```python
from build123d import *

# Parameters (mm, degrees)
F0_R     = 10.9982
F1_DEPTH = 7


with BuildPart() as f1:
    # F0 (on Top) → F1 (new body)
    with BuildSketch(Plane.XY):
        with BuildLine():
            ThreePointArc((12.246776, 8.324618), (12.094028, 24.483764), (14.8082, 40.414069))
            ThreePointArc((14.8082, 40.414069), (0, 55.222269), (-14.8082, 40.414069))
            ThreePointArc((-14.8082, 40.414069), (-12.094028, 24.483764), (-12.246776, 8.324618))
            ThreePointArc((-12.246776, 8.324618), (-12.824277, 7.4041), (-13.332719, 6.44371))
            ThreePointArc((-13.332719, 6.44371), (-27.250576, -1.768146), (-42.40371, -7.382757))
            ThreePointArc((-42.40371, -7.382757), (-47.823888, -27.611134), (-27.59551, -33.031312))
            ThreePointArc((-27.59551, -33.031312), (-15.156548, -22.715618), (-1.085942, -14.768328))
            ThreePointArc((-1.085942, -14.768328), (0, -14.8082), (1.085942, -14.768328))
            ThreePointArc((1.085942, -14.768328), (15.156548, -22.715618), (27.59551, -33.031312))
            ThreePointArc((27.59551, -33.031312), (47.823888, -27.611134), (42.40371, -7.382757))
            ThreePointArc((42.40371, -7.382757), (27.250576, -1.768146), (13.332719, 6.44371))
            ThreePointArc((13.332719, 6.44371), (12.824277, 7.4041), (12.246776, 8.324618))
        make_face()
        with Locations((-34.99961, -20.207034)):
            Circle(F0_R, mode=Mode.SUBTRACT)
        with Locations((34.99961, -20.207034)):
            Circle(F0_R, mode=Mode.SUBTRACT)
        Circle(F0_R, mode=Mode.SUBTRACT)
        with BuildLine():
            ThreePointArc((-10.9982, 40.414069), (0, 51.412269), (10.9982, 40.414069))
            ThreePointArc((10.9982, 40.414069), (0, 29.415869), (-10.9982, 40.414069))
        make_face(mode=Mode.SUBTRACT)
    extrude(amount=F1_DEPTH)


solid = f1.part
```
Geometry check sheet. Reference: the model listing, model coordinates, mm. A direction names the side the tool comes from. Coordinates: 2 decimals unless noted, no trailing zeros. Order: outer loops, then holes, each group sorted by start corner. A loop starts at its lowest first (then second) coordinate and runs counter-clockwise, first axis right, second up. Notation, with made-up numbers: (-13, 35) - (27, 35) arc R18 cw to (27, 43) - close; hole circle Ø8 at (71, 63.5). An arc over 180 degrees is marked (long way). Answer as a JSON object with one key per item and string values. Group by question number.
Item 1: Depth check by flat-ended pin: pin 1 Ø2 at (y, z) = (33, 3.5) entering from -X. Enter the tip coordinate at first touch or a pass-through.
Item 2: Scan lines: probe 1 along Y at (x, z) = (0, 5.75); probe 2 along X at (y, z) = (-22.5, 6.5); probe 3 along Y at (x, z) = (-9.5, 0.75). Record each from-to range of solid material in increasing order.
Item 3: Sectioned sample at B-B, the plane y = 0. Record the cut outline in (x, z), and give its area (3 significant figures).
Item 4: Sectioned sample at A-A, the plane x = 0. Record the cut outline in (y, z).
Item 5: Draft check along Y on faces 1 (the face through (-12.112, 24.71, 3.451)), 2 (the face through (45.49, -16.9, 3.45)), 3 (the face through (-11.3, 0.3, 0)), 4 (the face through (0.33, 55.22, 3.45)). Enter one of: +Y half, -Y half, draft (parallel to the pull), parting line (faces both ways), or undercut.
Item 6: Tool access check on faces 5 (the face through (-15.34, -22.84, 3.45)), 6 (the face through (-2.38, 51.15, 3.45)). Record the directions out of +Z, -Z, +X, -X, +Y, -Y that give a thin tool (end or side, any length) a straight path to the whole face; none if there is none.
Item 7: Sectioned sample at C-C, the plane x = -38. Record the cut outline in (y, z).
Resolved:
{
 "1": {"pin 1": "x = -13.36"},
 "2": {"probe 1": "-14.81 to -11, 11 to 29.42, 51.41 to 55.22", "probe 2": "-49.63 to -45.76, -24.24 to -14.84, 14.84 to 24.24, 45.76 to 49.63", "probe 3": "-19.12 to -5.54, 5.54 to 34.87, 45.96 to 51.77"},
 "3": {"outline": "(-23.73, 0) - (-11, 0) - (-11, 7) - (-23.73, 7) - close; (11, 0) - (23.73, 0) - (23.73, 7) - (11, 7) - close", "area": "178 mm^2"},
 "4": {"outline": "(-14.81, 0) - (-11, 0) - (-11, 7) - (-14.81, 7) - close; (11, 0) - (29.42, 0) - (29.42, 7) - (11, 7) - close; (51.41, 0) - (55.22, 0) - (55.22, 7) - (51.41, 7) - close"},
 "5": {"face 1": "undercut", "face 2": "undercut", "face 3": "draft", "face 4": "+Y half"},
 "6": {"face 5": "+Z, -Z, -Y", "face 6": "+Z, -Z"},
 "7": {"outline": "(-34.71, 0) - (-30.79, 0) - (-30.79, 7) - (-34.71, 7) - close; (-9.63, 0) - (-6.06, 0) - (-6.06, 7) - (-9.63, 7) - close"}
}
